Input: part model. Units: mm. Frame: model coordinates. Coordinates: 2 decimals unless noted, no trailing zeros. Loops run counter-clockwise (first coordinate to the right, second up) from the corner with the lowest first, then second, coordinate; pieces in that order, holes last.
Item 1: Section A-A on x = -23.03. Return loops of the section in (y, z), and give its area (3 significant figures).
Item 2: Ray query, line 1 along Y through (x, z) = (13.15, 0.8); line 2 along X through (y, z) = (15, 1); line 3 along X through (y, z) = (-14, 1.25). Return the intervals inside material, ascending.
Item 3: Section C-C on z = 1. Give the number of separate pieces and of enclosed holes in the cut face, and give its area (3 significant figures).
Item 4: Contact query for a flat-ended pin moving along its axis: P1, Ø2.5, axis at x = -23.03, y = -15, coming from the +Z side. Output: stop coordinate, or through.
Item 5: Section B-B on y = 15. Return loops of the section in (x, z), and give its area (3 significant figures).
```python
from build123d import *

# Parameters (mm, degrees)
SKETCH_1_W          = 84
SKETCH_1_H          = 36
EXTRUDE_1_DEPTH     = 2
SKETCH_2_R          = 1.5
CUT_EXTRUDE_1_DEPTH = 2


with BuildPart() as part:
    # 草图1 → 凸台-拉伸1 (new body)
    with BuildSketch(Plane.XY):
        Rectangle(SKETCH_1_W, SKETCH_1_H)
    extrude(amount=EXTRUDE_1_DEPTH)

    # 草图2 → 切除-拉伸1 (cut)
    with BuildSketch(Plane.XY.offset(2)):
        with Locations((23.15, -15)):
            Circle(SKETCH_2_R)
        with Locations((13.15, -15)):
            Circle(SKETCH_2_R)
        with Locations((-13.03, -15)):
            Circle(SKETCH_2_R)
        with Locations((-23.03, -15)):
            Circle(SKETCH_2_R)
        with Locations(Location((-23.03, 15, 0), (0, 0, 180))):
            Circle(SKETCH_2_R)
        with Locations(Location((-13.03, 15, 0), (0, 0, 180))):
            Circle(SKETCH_2_R)
        with Locations(Location((13.15, 15, 0), (0, 0, 180))):
            Circle(SKETCH_2_R)
        with Locations(Location((23.15, 15, 0), (0, 0, 180))):
            Circle(SKETCH_2_R)
    extrude(amount=-CUT_EXTRUDE_1_DEPTH, mode=Mode.SUBTRACT)


solid = part.part
```
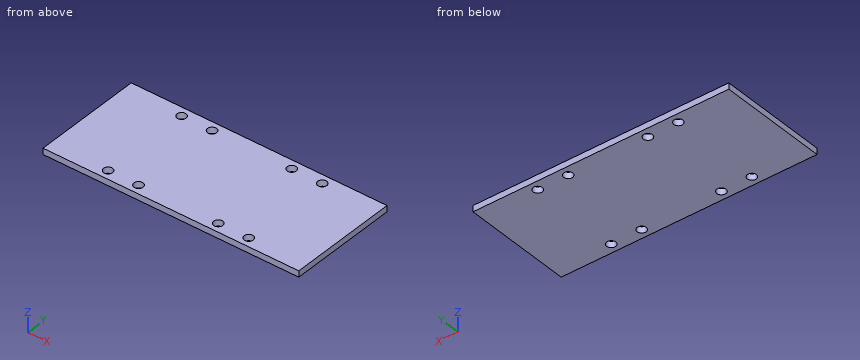
Results found:
1. outline: (-18, 0) - (-16.5, 0) - (-16.5, 2) - (-18, 2) - close; (-13.5, 0) - (13.5, 0) - (13.5, 2) - (-13.5, 2) - close; (16.5, 0) - (18, 0) - (18, 2) - (16.5, 2) - close
1. area: 60.0 mm2
2. line 1: y = -18 to -16.5, -13.5 to 13.5, 16.5 to 18
2. line 2: x = -42 to -24.53, -21.53 to -14.53, -11.53 to 11.65, 14.65 to 21.65, 24.65 to 42
2. line 3: x = -42 to -24.15, -21.91 to -14.15, -11.91 to 12.03, 14.27 to 22.03, 24.27 to 42
3. separate pieces: 1
3. enclosed holes: 8
3. area: 2,970 mm2
4. P1: passes through
5. outline: (-42, 0) - (-24.53, 0) - (-24.53, 2) - (-42, 2) - close; (-21.53, 0) - (-14.53, 0) - (-14.53, 2) - (-21.53, 2) - close; (-11.53, 0) - (11.65, 0) - (11.65, 2) - (-11.53, 2) - close; (14.65, 0) - (21.65, 0) - (21.65, 2) - (14.65, 2) - close; (24.65, 0) - (42, 0) - (42, 2) - (24.65, 2) - close
5. area: 144 mm2
